Read the model definition and answer for the solid it produces. Units are mm, in the model's axes. A direction names the side the tool comes from. Give positions to 0.01 mm unless a question says otherwise; leave off trailing zeros. Loops run counter-clockwise (first coordinate to the right, second up) from the corner with the lowest first, then second, coordinate; pieces in that order, holes last. Notation, with made-up numbers: (-11.75, 10.25) - (27.25, 10.25) arc R20 ccw to (27.25, 26.25) - close; hole circle Ø9 at (-35.5, -6). An arc over 180 degrees is marked (long way). Write item = value, one per line.
Autodesk Inventor part; units mm, degrees
ref_plane "YZ Plane" through (0, 0, 0) normal (1, 0, 0) x (0, 1, 0)
ref_plane "XZ Plane" through (0, 0, 0) normal (0, 1, 0) x (-1, 0, 0)
ref_plane "XY Plane" through (0, 0, 0) normal (0, 0, 1) x (1, 0, 0)
sketch "Sketch1" plane through (0, 0, 0) normal (0, 0, 1) x (1, 0, 0)
  line L0 (0, 0) -> (-29.8, 0)
  line L1 (0, 15.6035) -> (0, 0)
  circle A0 centre (-7.95, 7.8017) radius 5.95
  circle A1 centre (-21.85, 7.8017) radius 5.95
  line L2 (-29.8, 15.6035) -> (-29.8, 0)
  line L3 (-29.8, 15.6035) -> (0, 15.6035)
  line L4 (-29.8, 0) -> (-60, 0)
  line L5 (-21.85, 7.8017) -> (-21.85, 15.6035)
  line L6 (-21.85, 7.8017) -> (-21.85, 0)
  line L7 (-7.95, 7.8017) -> (-7.95, 0)
  line L8 (-7.95, 7.8017) -> (-7.95, 15.6035)
  line L9 (-59.6, 0) -> (-29.8, 0)
  line L10 (-59.6, 15.6035) -> (-59.6, 0)
  circle A2 centre (-51.65, 7.8017) radius 5.95
  circle A3 centre (-37.75, 7.8017) radius 5.95
  line L11 (-29.8, 15.6035) -> (-59.6, 15.6035)
  line L12 (-37.75, 7.8017) -> (-37.75, 15.6035)
  line L13 (-37.75, 7.8017) -> (-37.75, 0)
  line L14 (-51.65, 7.8017) -> (-51.65, 0)
  line L15 (-51.65, 7.8017) -> (-51.65, 15.6035)
  point P0 (0, 7.8017)
  point P1 (-59.6, 7.8017)
  dimension "d0" = 11.9
  dimension "d1" = 11.9
  dimension "d7" = 7.95
  dimension "d8" = 13.9
  dimension "d9" = 7.95
extrude "Extrusion1" add sketch "Sketch1" along normal blind 0.8 contours L0 L7 A0 L8 L3 L1 | L0 L6 A1 L5 L3 L8 A0 L7 | L0 L2 L3 L5 A1 L6 | L4 L13 A3 L12 L11 L2 | L4 L14 A2 L15 L11 L12 A3 L13 | L4 L10 L11 L15 A2 L14
sketch "Sketch2" plane through (0, 0, 0.8) normal (0, 0, 1) x (1, 0, 0)
  line L0 (-59.6, 15.6035) -> (-59.6, 0)
  line L1 (-59.6, 0) -> (0, 0)
  line L2 (-59.6, 15.6035) -> (0, 15.6035)
  line L3 (0, 15.6035) -> (0, 0)
  line L4 (0, 0) -> (-59.6, 0)
  line L5 (-59.6, 0) -> (-59.6, 15.6035)
extrude "Extrusion2" add sketch "Sketch2" along normal blind 6
sketch "Sketch3" plane through (-7.95, 7.8017, 0.8) normal (0, 0, -1) x (-1, 0, 0)
  circle A0 centre (0, 0) radius 5.95
  line L0 (0, 0) -> (-4.55, 0)
  line L1 (0, 0) -> (4.55, 0)
  line L2 (0, 0) -> (0, 4.55)
  line L3 (0, 0) -> (0, -4.55)
  line L4 (-4.55, 0) -> (-4.55, -1.8847)
  line L5 (0, 0) -> (2.5958, -2.5958)
  line L6 (0, 0) -> (3.671, 0) construction
  line L7 (3.2173, -3.2173) -> (-3.2173, 3.2173)
  line L8 (0, 0) -> (-3.2173, -3.2173)
  line L9 (0, 0) -> (3.2173, 3.2173)
  line L10 (-3.2173, -3.2173) -> (-1.8847, -4.55)
  line L11 (-3.2173, -3.2173) -> (-4.55, -1.8847)
  line L12 (3.2173, -3.2173) -> (1.8847, -4.55)
  line L13 (3.2173, -3.2173) -> (4.55, -1.8847)
  line L14 (4.55, 0) -> (4.55, -1.8847)
  line L15 (4.55, 0) -> (4.55, 1.8847)
  line L16 (3.2173, 3.2173) -> (4.55, 1.8847)
  line L17 (3.2173, 3.2173) -> (1.8847, 4.55)
  line L18 (0, 4.55) -> (1.8847, 4.55)
  line L19 (0, 4.55) -> (-1.8847, 4.55)
  line L20 (-3.2173, 3.2173) -> (-1.8847, 4.55)
  line L21 (-3.2173, 3.2173) -> (-4.55, 1.8847)
  line L22 (0, -4.55) -> (1.8847, -4.55)
  line L23 (0, -4.55) -> (-1.8847, -4.55)
  line L24 (-4.55, 0) -> (-4.55, 1.8847)
  line L25 (5.95, 0) -> (7.95, 0)
  circle A1 centre (13.9, 0) radius 5.95
  line L26 (6.95, 0) -> (6.95, 2.7112)
  line L27 (-7.95, 7.8017) -> (51.65, 7.8017)
  circle A2 centre (13.9, 0) radius 5.95
  line L28 (13.9, 0) -> (18.45, 0)
  line L29 (13.9, 0) -> (9.35, 0)
  line L30 (13.9, 0) -> (13.9, 4.55)
  line L31 (13.9, 0) -> (13.9, -4.55)
  line L32 (18.45, 0) -> (18.45, -1.8847)
  line L33 (13.9, 0) -> (11.3042, -2.5958)
  line L34 (13.9, 0) -> (10.229, 0) construction
  line L35 (10.6827, -3.2173) -> (17.1173, 3.2173)
  line L36 (13.9, 0) -> (17.1173, -3.2173)
  line L37 (13.9, 0) -> (10.6827, 3.2173)
  line L38 (17.1173, -3.2173) -> (15.7847, -4.55)
  line L39 (17.1173, -3.2173) -> (18.45, -1.8847)
  line L40 (10.6827, -3.2173) -> (12.0153, -4.55)
  line L41 (10.6827, -3.2173) -> (9.35, -1.8847)
  line L42 (9.35, 0) -> (9.35, -1.8847)
  line L43 (9.35, 0) -> (9.35, 1.8847)
  line L44 (10.6827, 3.2173) -> (9.35, 1.8847)
  line L45 (10.6827, 3.2173) -> (12.0153, 4.55)
  line L46 (13.9, 4.55) -> (12.0153, 4.55)
  line L47 (13.9, 4.55) -> (15.7847, 4.55)
  line L48 (17.1173, 3.2173) -> (15.7847, 4.55)
  line L49 (17.1173, 3.2173) -> (18.45, 1.8847)
  line L50 (13.9, -4.55) -> (12.0153, -4.55)
  line L51 (13.9, -4.55) -> (15.7847, -4.55)
  line L52 (18.45, 0) -> (18.45, 1.8847)
  line L53 (21.85, 7.8017) -> (21.85, -7.8017)
  line L54 (51.65, -7.8017) -> (-7.95, -7.8017)
  circle A3 centre (43.7, 0) radius 5.95
  line L55 (43.7, 0) -> (48.25, 0)
  line L56 (43.7, 0) -> (39.15, 0)
  line L57 (43.7, 0) -> (43.7, 4.55)
  line L58 (43.7, 0) -> (43.7, -4.55)
  line L59 (48.25, 0) -> (48.25, -1.8847)
  line L60 (43.7, 0) -> (41.1042, -2.5958)
  line L61 (43.7, 0) -> (40.029, 0) construction
  line L62 (40.4827, -3.2173) -> (46.9173, 3.2173)
  line L63 (43.7, 0) -> (46.9173, -3.2173)
  line L64 (43.7, 0) -> (40.4827, 3.2173)
  line L65 (46.9173, -3.2173) -> (45.5847, -4.55)
  line L66 (46.9173, -3.2173) -> (48.25, -1.8847)
  line L67 (40.4827, -3.2173) -> (41.8153, -4.55)
  line L68 (40.4827, -3.2173) -> (39.15, -1.8847)
  line L69 (39.15, 0) -> (39.15, -1.8847)
  line L70 (39.15, 0) -> (39.15, 1.8847)
  line L71 (40.4827, 3.2173) -> (39.15, 1.8847)
  line L72 (40.4827, 3.2173) -> (41.8153, 4.55)
  line L73 (43.7, 4.55) -> (41.8153, 4.55)
  line L74 (43.7, 4.55) -> (45.5847, 4.55)
  line L75 (46.9173, 3.2173) -> (45.5847, 4.55)
  line L76 (46.9173, 3.2173) -> (48.25, 1.8847)
  line L77 (43.7, -4.55) -> (41.8153, -4.55)
  line L78 (43.7, -4.55) -> (45.5847, -4.55)
  line L79 (48.25, 0) -> (48.25, 1.8847)
  line L80 (37.75, 0) -> (35.75, 0)
  circle A4 centre (29.8, 0) radius 5.95
  line L81 (36.75, 0) -> (36.75, 2.7112)
  line L82 (25.25, 0) -> (25.25, 1.8847)
  line L83 (25.25, 0) -> (25.25, -1.8847)
  line L84 (29.8, 0) -> (25.25, 0)
  line L85 (29.8, 0) -> (29.8, 4.55)
  line L86 (29.8, 0) -> (29.8, -4.55)
  line L87 (29.8, -4.55) -> (27.9153, -4.55)
  line L88 (29.8, 4.55) -> (31.6847, 4.55)
  line L89 (29.8, 0) -> (33.0173, 3.2173)
  line L90 (29.8, 0) -> (32.3958, -2.5958)
  line L91 (29.8, -4.55) -> (31.6847, -4.55)
  line L92 (33.0173, 3.2173) -> (34.35, 1.8847)
  line L93 (34.35, 0) -> (34.35, -1.8847)
  line L94 (33.0173, -3.2173) -> (26.5827, 3.2173)
  line L95 (33.0173, -3.2173) -> (34.35, -1.8847)
  circle A5 centre (29.8, 0) radius 5.95
  line L96 (33.0173, -3.2173) -> (31.6847, -4.55)
  line L97 (29.8, 0) -> (34.35, 0)
  line L98 (34.35, 0) -> (34.35, 1.8847)
  line L99 (29.8, 0) -> (33.471, 0) construction
  line L100 (26.5827, 3.2173) -> (27.9153, 4.55)
  line L101 (33.0173, 3.2173) -> (31.6847, 4.55)
  line L102 (29.8, 4.55) -> (27.9153, 4.55)
  line L103 (26.5827, 3.2173) -> (25.25, 1.8847)
  line L104 (26.5827, -3.2173) -> (25.25, -1.8847)
  line L105 (26.5827, -3.2173) -> (27.9153, -4.55)
  line L106 (29.8, 0) -> (26.5827, -3.2173)
  dimension "d14" = 4.55
  dimension "d15" = 4.55
  dimension "d16" = 4.55
  dimension "d17" = 4.55
  dimension "d22" = 45
sketch "Sketch4" plane through (-37.75, 7.8017, 0.8) normal (0, 0, -1) x (-1, 0, 0)
  line L0 (3.2173, -3.2173) -> (1.8847, -4.55)
  line L1 (3.2173, -3.2173) -> (4.55, -1.8847)
  line L2 (4.55, 0) -> (4.55, -1.8847)
  line L3 (4.55, 0) -> (4.55, 1.8847)
  line L4 (3.2173, 3.2173) -> (4.55, 1.8847)
  line L5 (3.2173, 3.2173) -> (1.8847, 4.55)
  line L6 (0, 4.55) -> (1.8847, 4.55)
  line L7 (0, 4.55) -> (-1.8847, 4.55)
  line L8 (-3.2173, 3.2173) -> (-1.8847, 4.55)
  line L9 (-3.2173, 3.2173) -> (-4.55, 1.8847)
  line L10 (-4.55, 0) -> (-4.55, 1.8847)
  line L11 (-4.55, 0) -> (-4.55, -1.8847)
  line L12 (-3.2173, -3.2173) -> (-4.55, -1.8847)
  line L13 (-3.2173, -3.2173) -> (-1.8847, -4.55)
  line L14 (0, -4.55) -> (-1.8847, -4.55)
  line L15 (0, -4.55) -> (1.8847, -4.55)
  line L16 (-4.55, 1.8847) -> (-4.55, -1.8847)
  line L17 (-1.8847, -4.55) -> (1.8847, -4.55)
  line L18 (4.55, -1.8847) -> (4.55, 1.8847)
  line L19 (1.8847, 4.55) -> (-1.8847, 4.55)
  line L20 (1.8847, -4.55) -> (4.55, -1.8847)
  line L21 (-1.8847, -4.55) -> (-4.55, -1.8847)
  line L22 (-4.55, 1.8847) -> (-1.8847, 4.55)
  line L23 (1.8847, 4.55) -> (4.55, 1.8847)
  circle A0 centre (0, 0) radius 5.95
  circle A1 centre (0, 0) radius 5.95
  line L24 (10.6827, 3.2173) -> (12.0153, 4.55)
  line L25 (10.6827, 3.2173) -> (9.35, 1.8847)
  line L26 (9.35, 0) -> (9.35, 1.8847)
  line L27 (9.35, 0) -> (9.35, -1.8847)
  line L28 (10.6827, -3.2173) -> (9.35, -1.8847)
  line L29 (10.6827, -3.2173) -> (12.0153, -4.55)
  line L30 (13.9, -4.55) -> (12.0153, -4.55)
  line L31 (13.9, -4.55) -> (15.7847, -4.55)
  line L32 (17.1173, -3.2173) -> (15.7847, -4.55)
  line L33 (17.1173, -3.2173) -> (18.45, -1.8847)
  line L34 (18.45, 0) -> (18.45, -1.8847)
  line L35 (18.45, 0) -> (18.45, 1.8847)
  line L36 (17.1173, 3.2173) -> (18.45, 1.8847)
  line L37 (17.1173, 3.2173) -> (15.7847, 4.55)
  line L38 (13.9, 4.55) -> (15.7847, 4.55)
  line L39 (13.9, 4.55) -> (12.0153, 4.55)
  line L40 (9.35, 1.8847) -> (12.0153, 4.55)
  line L41 (12.0153, 4.55) -> (15.7847, 4.55)
  line L42 (15.7847, 4.55) -> (18.45, 1.8847)
  line L43 (18.45, 1.8847) -> (18.45, -1.8847)
  line L44 (18.45, -1.8847) -> (15.7847, -4.55)
  line L45 (9.35, -1.8847) -> (12.0153, -4.55)
  line L46 (-15.9, 4.55) -> (-17.7847, 4.55)
  line L47 (-15.9, 4.55) -> (-14.0153, 4.55)
  line L48 (-12.6827, 3.2173) -> (-14.0153, 4.55)
  line L49 (-12.6827, 3.2173) -> (-11.35, 1.8847)
  line L50 (-11.35, 0) -> (-11.35, 1.8847)
  line L51 (-11.35, 0) -> (-11.35, -1.8847)
  line L52 (-12.6827, -3.2173) -> (-11.35, -1.8847)
  line L53 (-12.6827, -3.2173) -> (-14.0153, -4.55)
  line L54 (-15.9, -4.55) -> (-14.0153, -4.55)
  line L55 (-15.9, -4.55) -> (-17.7847, -4.55)
  line L56 (-19.1173, -3.2173) -> (-17.7847, -4.55)
  line L57 (-19.1173, -3.2173) -> (-20.45, -1.8847)
  line L58 (-20.45, 0) -> (-20.45, -1.8847)
  line L59 (-20.45, 0) -> (-20.45, 1.8847)
  line L60 (-19.1173, 3.2173) -> (-20.45, 1.8847)
  line L61 (-19.1173, 3.2173) -> (-17.7847, 4.55)
  line L62 (-17.7847, 4.55) -> (-14.0153, 4.55)
  line L63 (-11.35, 1.8847) -> (-14.0153, 4.55)
  line L64 (-17.7847, 4.55) -> (-20.45, 1.8847)
  line L65 (-20.45, -1.8847) -> (-17.7847, -4.55)
  line L66 (-17.7847, -4.55) -> (-14.0153, -4.55)
  line L67 (-11.35, -1.8847) -> (-11.35, 1.8847)
  line L68 (-11.35, -1.8847) -> (-14.0153, -4.55)
  circle A2 centre (-15.9, 0) radius 5.95
  line L69 (-33.0173, 3.2173) -> (-34.35, 1.8847)
  line L70 (-33.0173, 3.2173) -> (-31.6847, 4.55)
  line L71 (-29.8, 4.55) -> (-31.6847, 4.55)
  line L72 (-29.8, 4.55) -> (-27.9153, 4.55)
  line L73 (-26.5827, 3.2173) -> (-27.9153, 4.55)
  line L74 (-26.5827, 3.2173) -> (-25.25, 1.8847)
  line L75 (-25.25, 0) -> (-25.25, 1.8847)
  line L76 (-25.25, 0) -> (-25.25, -1.8847)
  line L77 (-26.5827, -3.2173) -> (-25.25, -1.8847)
  line L78 (-26.5827, -3.2173) -> (-27.9153, -4.55)
  line L79 (-29.8, -4.55) -> (-27.9153, -4.55)
  line L80 (-29.8, -4.55) -> (-31.6847, -4.55)
  line L81 (-33.0173, -3.2173) -> (-31.6847, -4.55)
  line L82 (-33.0173, -3.2173) -> (-34.35, -1.8847)
  line L83 (-34.35, 0) -> (-34.35, -1.8847)
  line L84 (-34.35, 1.8847) -> (-31.6847, 4.55)
  line L85 (-27.9153, 4.55) -> (-25.25, 1.8847)
  line L86 (-25.25, -1.8847) -> (-27.9153, -4.55)
  line L87 (-31.6847, -4.55) -> (-27.9153, -4.55)
  line L88 (-34.35, -1.8847) -> (-31.6847, -4.55)
  line L89 (-34.35, -1.8847) -> (-34.35, 1.8847)
  circle A3 centre (-29.8, 0) radius 5.95
  circle A4 centre (13.9, 0) radius 5.95
  circle A5 centre (13.9, 0) radius 5.95
  line L90 (-31.6847, 4.55) -> (-27.9153, 4.55)
  line L91 (-25.25, 1.8847) -> (-25.25, -1.8847)
  line L92 (-20.45, -1.8847) -> (-20.45, 1.8847)
  line L93 (9.35, -1.8847) -> (9.35, 1.8847)
  line L94 (12.0153, -4.55) -> (15.7847, -4.55)
  point P0 (-37.75, -7.8017)
extrude "Extrusion3" cut sketch "Sketch4" against normal blind 1.5 contours L0 L15 L14 L13 L12 L11 L10 L9 L8 L7 L6 L5 L4 L3 L2 L1 | L24 L39 L38 L37 L36 L35 L34 L33 L32 L31 L30 L29 L28 L27 L26 L25 | L47 L48 L49 L50 L51 L52 L53 L54 L55 L56 L57 L58 L59 L60 L61 L46 | L70 L71 L72 L73 L74 L75 L76 L77 L78 L79 L80 L81 L82 L83 L89 L69
sketch "Sketch5" plane through (-37.75, 7.8017, 2.3) normal (0, 0, -1) x (-1, 0, 0)
  circle A0 centre (0, 0) radius 3.1
  circle A1 centre (0, 0) radius 3.1
  circle A2 centre (13.9, 0) radius 3.1
  circle A3 centre (-15.9, 0) radius 3.1
  circle A4 centre (-29.8, 0) radius 3.1
  line L0 (-25.25, 1.8847) -> (-25.25, -1.8847)
  line L1 (-34.35, -1.8847) -> (-34.35, 1.8847)
  line L2 (-25.25, -1.8847) -> (-27.9153, -4.55)
  circle A5 centre (-29.8, 0) radius 4.9249
  line L3 (-15.9, 0) -> (-20.45, 0)
  line L4 (-20.45, -1.8847) -> (-20.45, 1.8847)
  line L5 (-15.9, 0) -> (-11.35, 0)
  line L6 (-11.35, 1.8847) -> (-11.35, -1.8847)
  line L7 (0, 0) -> (-4.55, 0)
  line L8 (-4.55, -1.8847) -> (-4.55, 1.8847)
  line L9 (0, 0) -> (4.55, 0)
  line L10 (4.55, 1.8847) -> (4.55, -1.8847)
  line L11 (13.9, 0) -> (9.35, 0)
  line L12 (9.35, -1.8847) -> (9.35, 1.8847)
  line L13 (18.45, 1.8847) -> (18.45, -1.8847)
  line L14 (18.45, 0) -> (13.9, 0)
  point P0 (-37.75, -7.8017)
  dimension "d25" = 6.2
  dimension "d26" = 6.2
  dimension "d27" = 6.2
  dimension "d28" = 6.2
  dimension "d29" = 6.2
extrude "Extrusion4" cut sketch "Sketch5" against normal through all contours L9 L7 A0 | A0 L7 L9 | L14 L11 A2 | A2 L11 L14 | L5 L3 A3 | A3 L3 L5 | A4
properties part number "switch_mount"
1) A cutting plane is placed at C-C on x = -53. Determine the outline of the cut face in (y, z), then the cut area to 3 significant figures.
Output:
outline = (0, 0) - (2.01, 0) - (2.01, 0.8) - (3.25, 0.8) - (3.25, 2.3) - (5.01, 2.3) - (5.01, 6.8) - (0, 6.8) - close; (10.59, 2.3) - (12.35, 2.3) - (12.35, 0.8) - (13.6, 0.8) - (13.6, 0) - (15.6, 0) - (15.6, 6.8) - (10.59, 6.8) - close
area = 58.1 mm²
2) A tool of negligible diameter and unlimited length cuts with its end or side. For faces 4 (the face through (-30, 8, 6.8)), 5 (the face through (-8, 12.352, 2)), from which of +Z, -Z, +X, -X, +Y, -Y can it reach the whole face along a straight path? Write none if from no direction.
Output:
face_4 = +Z, +X, -X, +Y, -Y
face_5 = -Z
3) The mould has two halves that part along Y. Classify faces 1 (the face through (-30, 0, 3)), 2 (the face through (-48.6, 11.4, 0.8)), 3 (the face through (-30, 8, 0)): pulls with the +Y half, pulls with the -Y half, needs draft (parallel to the pull), parting line crosses it, or undercut.
Output:
face_1 = pulls with the -Y half
face_2 = undercut
face_3 = needs draft
4) Find the intervals of material crossed by probe 1 along X at (y, z) = (7.75, 4.5); probe 2 along X at (y, z) = (7, 2); probe 3 along Y at (x, z) = (-51.65, 4.05), in increasing order.
Output:
probe_1 = -59.6 to -54.75, -48.55 to -40.85, -34.65 to -24.95, -18.75 to -11.05, -4.85 to 0
probe_2 = -59.6 to -56.2, -47.1 to -42.3, -33.2 to -26.4, -17.3 to -12.5, -3.4 to 0
probe_3 = 0 to 4.7, 10.9 to 15.6
5) A cutting plane is placed at B-B on z = 5. Determine the outline of the cut face in (x, y), then the cut area to 3 significant figures.
Output:
outline = (-59.6, 0) - (0, 0) - (0, 15.6) - (-59.6, 15.6) - close; hole circle Ø6.2 at (-51.65, 7.8); hole circle Ø6.2 at (-37.75, 7.8); hole circle Ø6.2 at (-21.85, 7.8); hole circle Ø6.2 at (-7.95, 7.8)
area = 809 mm²
6) A cutting plane is placed at A-A on x = -37.75. Determine the outline of the cut face in (y, z).
Output:
outline = (0, 0) - (1.85, 0) - (1.85, 0.8) - (3.25, 0.8) - (3.25, 2.3) - (4.7, 2.3) - (4.7, 6.8) - (0, 6.8) - close; (10.9, 2.3) - (12.35, 2.3) - (12.35, 0.8) - (13.75, 0.8) - (13.75, 0) - (15.6, 0) - (15.6, 6.8) - (10.9, 6.8) - close
7) This flat-tipped pin is pushed along its axis until it touches: P1, Ø2.5, axis at x = -9.5, y = 6.5, coming from the -Z side. Where does it stop, or does it pass through?
Output:
P1 = 2.3
8) A cutting plane is placed at D-D on y = 6.5. Give the number of separate pieces and of enclosed holes in the cut face, then the cut area to 3 significant figures.
Output:
separate_pieces = 5
enclosed_holes = 0
area = 212 mm²
